Autodesk Inventor part; units mm, degrees
ref_plane "YZ Plane" through (0, 0, 0) normal (1, 0, 0) x (0, 1, 0)
ref_plane "XZ Plane" through (0, 0, 0) normal (0, 1, 0) x (-1, 0, 0)
ref_plane "XY Plane" through (0, 0, 0) normal (0, 0, 1) x (1, 0, 0)
sketch "Sketch1" plane through (0, 0, 0) normal (0, 0, 1) x (1, 0, 0)
  circle A0 centre (-14.45, 0) radius 0.6
  line L0 (-14.45, 0) -> (23.65, 0) construction
  line L1 (-14.45, -3.175) -> (23.65, -3.175)
  line L2 (23.65, 3.175) -> (-14.45, 3.175)
  arc A1 (-14.45, 3.175) -> (-14.45, -3.175) centre (-14.45, 0) ccw
  arc A2 (23.65, -3.175) -> (23.65, 3.175) centre (23.65, 0) ccw
  line L3 (-14.45, 0) -> (23.65, 0) construction
  circle A3 centre (23.65, 0) radius 6.35
  point P0 (0, 0)
  point P1 (4.6, 0)
  point P2 (18.1507, -3.175)
  point P3 (18.1507, 3.175)
  dimension "d0" = 38.1
  dimension "d1" = 0
  dimension "d2" = 6.35
  dimension "d3" = 12.7
extrude "Extrusion1" add sketch "Sketch1" along normal blind 2.54
properties part number "ShutterStop"
Source: CAD feature listing. Evaluate the final solid. Frame: model axes, mm. A direction names the side the tool comes from. Give positions to 0.01 mm unless a question says otherwise; leave off trailing zeros. Order: outer loops, then holes, each group sorted by start corner. A loop starts at its lowest first (then second) coordinate and runs counter-clockwise, first axis right, second up. Notation, with made-up numbers: (89.25, 54.5) -> (146.25, 54.5) arc R25 ccw to (146.25, 79.5) -> close; hole circle Ø6 at (80.25, 72.25). An arc over 180 degrees is marked (long way). Write item = value, one per line.
Q1. Cut plane B-B, the plane z = 0.55. Output: boundary loops of the cut face in (x, y) (3 decimals).
Data:
outline = (-14.45, -3.175) -> (18.151, -3.175) arc R6.35 ccw (long way) to (18.151, 3.175) -> (-14.45, 3.175) arc R3.175 ccw to start; hole circle Ø1.2 at (-14.45, 0)
Q2. Set-up query: faces 5 (the face through (2, -3.175, 1)), 6 (the face through (6, 0, 0)). Return all of +Z, -Z, +X, -X, +Y, -Y with unobstructed straight access to the full face (end or side cutting, diameter ignored); none if empty.
Data:
face_5 = +Z, -Z, -X, -Y
face_6 = -Z, +X, -X, +Y, -Y
Q3. Material intervals for line 1 (Y direction, x = -14.45, z = 0.5) (3 decimals); line 2 (Y direction, x = -13.5, z = 1.3) (3 decimals); line 3 (X direction, y = 0.5, z = 2), sorted ascending. Write a range as from..to.
Data:
line_1 = -3.175..-0.6, 0.6..3.175
line_2 = -3.175..3.175
line_3 = -17.59..-14.78, -14.12..29.98
Q4. Pull-direction query (X, two-part tool) for faces 1 (the face through (30, 0, 1)), 2 (the face through (-13.896, 0.23, 1.252)), 3 (the face through (2, 3.175, 1)), 4 (the face through (-17.624, -0.07, 1.252)); classes: released by +X, released by -X, zero draft, split by the parting line, or undercut.
Data:
face_1 = split by the parting line
face_2 = undercut
face_3 = zero draft
face_4 = released by -X
Q5. Cut plane A-A, the plane y = 0. Output: boundary loops of the cut face in (x, z) (3 decimals), and give its area (3 significant figures).
Data:
outline = (-17.625, 0) -> (-15.05, 0) -> (-15.05, 2.54) -> (-17.625, 2.54) -> close; (-13.85, 0) -> (30, 0) -> (30, 2.54) -> (-13.85, 2.54) -> close
area = 118 mm^2
Q6. Cut plane C-C, the plane x = -10. Output: boundary loops of the cut face in (y, z) (3 decimals).
Data:
outline = (-3.175, 0) -> (3.175, 0) -> (3.175, 2.54) -> (-3.175, 2.54) -> close
Q7. Pin query (flat end, axial travel): pin 1 (1.5 mm diameter, centred on y = -3, z = 2, fed in from +X); pin 2 (1.5 mm diameter, centred on x = 7.5, z = 1, fed in from +Y) (3 decimals). Return the tip coordinate at first contact, or that it passes through.
Data:
pin_1 = 29.59
pin_2 = 3.175
Q8. Cut plane D-D, the plane y = -2.25. Output: boundary loops of the cut face in (x, z), and give its area (3 significant figures).
Data:
outline = (-16.69, 0) -> (29.59, 0) -> (29.59, 2.54) -> (-16.69, 2.54) -> close
area = 118 mm^2
